Build history of the part. All positions in model axes, mm. Face numbers are marked on the shaded views. Round coordinates to 2 decimals unless told otherwise and drop trailing zeros. Order: outer loops, then holes, each group sorted by start corner. A loop starts at its lowest first (then second) coordinate and runs counter-clockwise, first axis right, second up. Notation, with made-up numbers: (-4.75, 50) - (-0.75, 50) arc R24 ccw to (-0.75, 65) - close; hole circle Ø5 at (53.25, -39). An arc over 180 degrees is marked (long way). One line per question, with ' | ' between items. Start each with the question number.
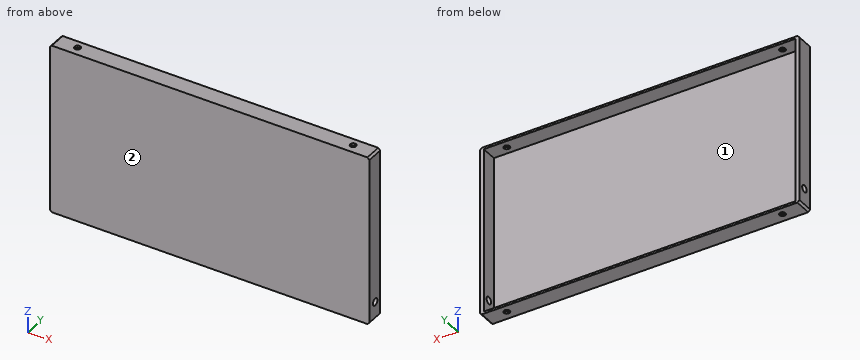
from build123d import *

# Parameters (mm, degrees)
SKETCH1_W           = 160
SKETCH1_H           = 85
BOSS_EXTRUDE1_DEPTH = 0.6
SKETCH2_W           = 160
SKETCH2_H           = 85
SKETCH2_W_2         = 156
SKETCH2_H_2         = 82.875
BOSS_EXTRUDE2_DEPTH = 8
CHAMFER1_SIZE       = 1
SKETCH3_R           = 1.5
CUT_EXTRUDE1_DEPTH  = 98
SKETCH4_R           = 1.75
CUT_EXTRUDE2_DEPTH  = 1000


with BuildPart() as part:
    # Sketch1 → Boss-Extrude1 (new body)
    with BuildSketch(Plane(origin=(0, 0, 0), x_dir=(1, 0, 0), z_dir=(0, 1, 0))):
        Rectangle(SKETCH1_W, SKETCH1_H)
    extrude(amount=BOSS_EXTRUDE1_DEPTH)

    # Sketch2 → Boss-Extrude2 (add)
    with BuildSketch(Plane(origin=(0, 0.6, 0), x_dir=(1, 0, 0), z_dir=(0, 1, 0))):
        Rectangle(SKETCH2_W, SKETCH2_H)
        Rectangle(SKETCH2_W_2, SKETCH2_H_2, mode=Mode.SUBTRACT)
    extrude(amount=BOSS_EXTRUDE2_DEPTH)

    # Chamfer1
    chamfer1_edges = [part.edges().sort_by_distance(p)[0] for p in [
        (80, 4.3, 42.5),
        (-80, 4.3, 42.5),
        (-80, 4.3, -42.5),
        (80, 4.3, -42.5),
    ]]
    chamfer(chamfer1_edges, length=CHAMFER1_SIZE)

    # Sketch3 → Cut-Extrude1 (cut)
    with BuildSketch(Plane.XY.offset(42.5)):
        with Locations((-69, 4.6)):
            Circle(SKETCH3_R)
        with Locations((69, 4.6)):
            Circle(SKETCH3_R)
    extrude(amount=-CUT_EXTRUDE1_DEPTH, mode=Mode.SUBTRACT)

    # Sketch4 → Cut-Extrude2 (cut)
    with BuildSketch(Plane(origin=(80, 0, 0), x_dir=(0, 0, -1), z_dir=(1, 0, 0))):
        with Locations((33.5, 4.6)):
            Circle(SKETCH4_R)
    extrude(amount=-CUT_EXTRUDE2_DEPTH, mode=Mode.SUBTRACT)


solid = part.part
Item 1: Pull direction Z, two halves, no side cores. Call the marked faces 1 and 2: released by +Z, released by -Z, zero draft, split by the parting line, or undercut.
Item 2: Wall check: line 1 along X through (y, z) = (3.25, -15); line 2 along Y through (x, z) = (-69, 41.85); line 3 along Z through (x, y) = (58, 6.75). Give the ranges that are in metal, low to high. Write a range as [from, to].
Item 3: Slice it at C-C (z = -1.5). Write the cut outline in (x, y).
Item 4: Slice it at B-B (x = -69). Write the cut outline in (y, z), plus the area to 3 significant figures.
Item 5: Slice it at D-D (x = 16). Write the cut outline in (y, z).
Item 6: Slice it at A-A (z = -33.5). Write the cut outline in (x, y), plus the area to 3 significant figures.
Item 7: Pin check, flat tip, straight feed: pin 1 (4 mm diameter, centred on x = -40.5, z = 9, fed in from +Y). Stop position of the tip, or through.
A:
1) face 1: undercut | face 2: zero draft
2) line 1: [-80, -78], [78, 80] | line 2: [0, 3.1], [6.1, 8.6] | line 3: [-42.5, -41.44], [41.44, 42.5]
3) outline: (-80, 0) - (80, 0) - (80, 8.6) - (78, 8.6) - (78, 0.6) - (-78, 0.6) - (-78, 8.6) - (-80, 8.6) - close
4) outline: (0, -42.5) - (3.1, -42.5) - (3.1, -41.44) - (0.6, -41.44) - (0.6, 41.44) - (3.1, 41.44) - (3.1, 42.5) - (0, 42.5) - close; (6.1, -42.5) - (8.6, -42.5) - (8.6, -41.44) - (6.1, -41.44) - close; (6.1, 41.44) - (8.6, 41.44) - (8.6, 42.5) - (6.1, 42.5) - close | area: 61.6 mm^2
5) outline: (0, -42.5) - (8.6, -42.5) - (8.6, -41.44) - (0.6, -41.44) - (0.6, 41.44) - (8.6, 41.44) - (8.6, 42.5) - (0, 42.5) - close
6) outline: (-80, 0) - (80, 0) - (80, 2.85) - (78, 2.85) - (78, 0.6) - (-78, 0.6) - (-78, 2.85) - (-80, 2.85) - close; (-80, 6.35) - (-78, 6.35) - (-78, 8.6) - (-80, 8.6) - close; (78, 6.35) - (80, 6.35) - (80, 8.6) - (78, 8.6) - close | area: 114 mm^2
7) pin 1: y = 0.6
